from build123d import *

# Parameters (mm, degrees)
SKETCH2_R           = 16.37540157
SKETCH2_W           = 30
SKETCH2_H           = 50
SKETCH2_W_2         = 16.72757971
SKETCH2_H_2         = 91.338041812
BOSS_EXTRUDE1_DEPTH = 8
CUT_EXTRUDE1_DEPTH  = 3
SKETCH7_W           = 21
SKETCH7_H           = 41
SKETCH7_W_2         = 7
SKETCH7_H_2         = 18
CUT_EXTRUDE2_DEPTH  = 97.732382254
SKETCH8_W           = 42.713825064
SKETCH8_H           = 72.244370788
CUT_EXTRUDE3_DEPTH  = 97.732382254
SKETCH10_W          = 16.72757971
SKETCH10_H          = 8
BOSS_EXTRUDE3_DEPTH = 43
CUT_EXTRUDE4_DEPTH  = 23
SKETCH12_W          = 9.409731529
SKETCH12_H          = 26.743509799
SKETCH12_W_2        = 7.397521328
SKETCH12_H_2        = 21.048617388
CUT_EXTRUDE5_DEPTH  = 10


with BuildPart() as part:
    # Sketch2 → Boss-Extrude1 (new body)
    with BuildSketch(Plane(origin=(0, 0, 0), x_dir=(1, 0, 0), z_dir=(0, 1, 0))):
        with Locations((0, -45.669020906)):
            Circle(SKETCH2_R)
        with Locations((0, 70)):
            Rectangle(SKETCH2_W, SKETCH2_H)
        Rectangle(SKETCH2_W_2, SKETCH2_H_2)
    extrude(amount=BOSS_EXTRUDE1_DEPTH)

    # Sketch6 → Cut-Extrude1 (cut)
    with BuildSketch(Plane(origin=(0, 8, 0), x_dir=(1, 0, 0), z_dir=(0, 1, 0))):
        with BuildLine():
            Line((-2.999771067, 18.037061373), (-4.97435622, 4.183990942))
            ThreePointArc((-4.97435622, 4.183990942), (0, -6.5), (4.97435622, 4.183990942))
            Line((4.97435622, 4.183990942), (2.999771067, 18.037061373))
            ThreePointArc((2.999771067, 18.037061373), (0, 21), (-2.999771067, 18.037061373))
        make_face()
    extrude(amount=-CUT_EXTRUDE1_DEPTH, mode=Mode.SUBTRACT)

    # Sketch7 → Cut-Extrude2 (cut, through all)
    with BuildSketch(Plane.XZ):
        with Locations((0, -70)):
            Rectangle(SKETCH7_W, SKETCH7_H)
        with Locations((0, -49.5)):
            Rectangle(SKETCH7_W_2, SKETCH7_H_2)
    extrude(amount=-CUT_EXTRUDE2_DEPTH, mode=Mode.SUBTRACT)

    # Sketch8 → Cut-Extrude3 (cut, through all)
    with BuildSketch(Plane.XZ):
        with Locations((-1.974672585, -63.480825527)):
            Rectangle(SKETCH8_W, SKETCH8_H)
    extrude(amount=-CUT_EXTRUDE3_DEPTH, mode=Mode.SUBTRACT)

    # Sketch10 → Boss-Extrude3 (add)
    with BuildSketch(Plane(origin=(0, 0, -27.358640133), x_dir=(-1, 0, 0), z_dir=(0, 0, -1))):
        with Locations((0, 4)):
            Rectangle(SKETCH10_W, SKETCH10_H)
    extrude(amount=BOSS_EXTRUDE3_DEPTH)

    # Sketch11 → Cut-Extrude4 (cut)
    with BuildSketch(Plane.XZ):
        Polygon((-8.363789855, -58.228971018), (0, -70.358640133), (8.363789855, -58.228971018), (14.634786806, -58.228971018), (14.634786806, -78.124340067), (-16.486460869, -78.124340067), (-15.81957699, -58.228971018), align=None)
    extrude(amount=-CUT_EXTRUDE4_DEPTH, mode=Mode.SUBTRACT)

    # Sketch12 → Cut-Extrude5 (cut)
    with BuildSketch(Plane(origin=(0, 8, 0), x_dir=(1, 0, 0), z_dir=(0, 1, 0))):
        with Locations((0.538728684, 43.496138516)):
            Rectangle(SKETCH12_W, SKETCH12_H)
        with Locations((0.054120037, -21.966665665)):
            Rectangle(SKETCH12_W_2, SKETCH12_H_2)
        with BuildLine():
            ThreePointArc((3.752880701, -32.490974359), (0.054120037, -45.382739126), (-3.644640627, -32.490974359))
            Line((-3.644640627, -32.490974359), (3.752880701, -32.490974359))
        make_face()
        Polygon((5.243594448, 56.867893415), (1.087937996, 63.395652597), (-4.166137081, 56.867893415), align=None)
    extrude(amount=-CUT_EXTRUDE5_DEPTH, mode=Mode.SUBTRACT)


solid = part.part
Here's how the part is built. I have some questions about the finished solid (model axes, mm). A direction names the side the tool comes from. Coordinates: 2 decimals unless noted, no trailing zeros. Write each loop counter-clockwise with the first axis right and the second up, starting at its lowest first coordinate (ties: lowest second). Pieces come first, ordered by that corner, then holes.
1) If we section it at C-C (z = 0): List the corners of the cut face in (x, y) for me, plus the area to 3 significant figures.
Filled in:
outline: (-8.36, 0) - (8.36, 0) - (8.36, 8) - (6.5, 8) - (6.5, 5) - (-6.5, 5) - (-6.5, 8) - (-8.36, 8) - close
area: 94.8 mm2
2) I'm going to push flat-ended pins straight in: pin 1 (1.5 mm diameter, centred on y = 3, z = 3, fed in from +X); pin 2 (18 mm diameter, centred on x = 0.05, z = 38.41, fed in from +Y); pin 3 (3 mm diameter, centred on x = -6, y = 5.5, fed in from -Z); pin 4 (3 mm diameter, centred on y = 5, z = -54.5, fed in from -X). Where does each tip first touch, or does it pass through?
Filled in:
pin 1: stops at x = 8.36
pin 2: stops at y = 8
pin 3: stops at z = -63.83
pin 4: stops at x = -8.36
3) If we section it at B-B (y = 6.75): List the corners of the cut face in (x, z) for me.
Filled in:
outline: (-8.36, -58.23) - (0, -70.36) - (8.36, -58.23) - (8.36, 31.59) arc R16.38 ccw (long way) to (-8.36, 31.59) - close; hole (-4.97, -4.18) - (-3, -18.04) arc R3 ccw to (3, -18.04) - (4.97, -4.18) arc R6.5 ccw (long way) to start; hole (-4.17, -56.87) - (1.09, -63.4) - (5.24, -56.87) - (5.24, -30.12) - (-4.17, -30.12) - close; hole (-3.64, 11.44) - (3.75, 11.44) - (3.75, 32.49) arc R6.98 ccw (long way) to (-3.64, 32.49) - close
4) If we section it at A-A (z = -45.5): List the corners of the cut face in (x, y) for me, plus the area to 3 significant figures.
Filled in:
outline: (-8.36, 0) - (-4.17, 0) - (-4.17, 8) - (-8.36, 8) - close; (5.24, 0) - (8.36, 0) - (8.36, 8) - (5.24, 8) - close
area: 58.5 mm2
5) If we section it at D-D (z = 20): List the corners of the cut face in (x, y) for me, plus the area to 3 significant figures.
Filled in:
outline: (-8.36, 0) - (-3.64, 0) - (-3.64, 8) - (-8.36, 8) - close; (3.75, 0) - (8.36, 0) - (8.36, 8) - (3.75, 8) - close
area: 74.6 mm2
6) Thinking about a two-plate mould opening in X: for faces 4 (the face through (4, 0, 11)), 5 (the face through (-4.166, 4, -43)), 6 (the face through (4.123, 3.944, -64.379)), which applies, +X half, -X half, draft (parallel to the pull), parting line (faces both ways), or undercut?
Filled in:
face 4: draft
face 5: undercut
face 6: +X half
7) Which directions (+Z, -Z, +X, -X, +Y, -Y) give clear straight access to the entire face, cutting with the end or side of a thin tool? Please do faces 1 (the face through (0, 5, -4)), 2 (the face through (-8.364, 4, -13)), 3 (the face through (-3.645, 4, 22)).
Filled in:
face 1: +Y
face 2: -Z, -X, +Y, -Y
face 3: +Y, -Y
8) If I drill on line 1 (X direction, y = 5.5, z = -56); line 2 (X direction, y = 7.35, z = 0); line 3 (Z direction, x = 2, y = 3), over which ranges is the centre line in solid material (lowest first)?
Filled in:
line 1: x = -8.36 to -4.17, 5.24 to 8.36
line 2: x = -8.36 to -6.5, 6.5 to 8.36
line 3: z = -67.46 to -61.96, -30.12 to 11.44, 45.11 to 61.92
